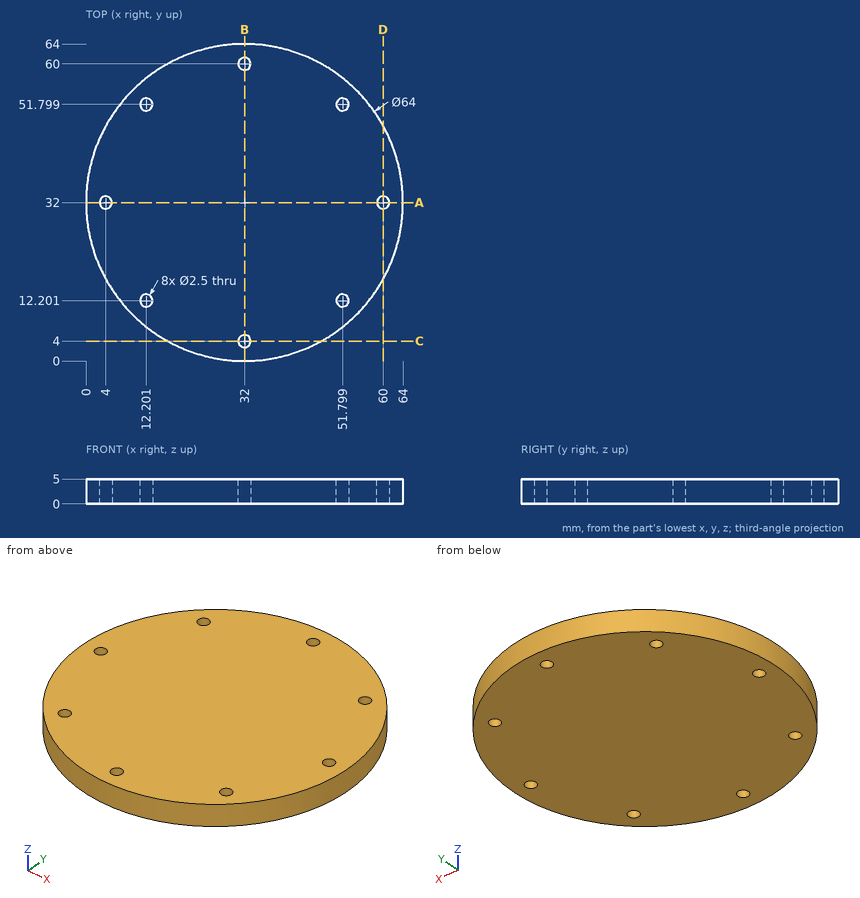
For this review, use the dimensioned drawing (mm, ordinates from the lowest corner) and the shaded views. Give positions to 0.01 mm unless a question says otherwise; leave off trailing zeros. Loops run counter-clockwise (first coordinate to the right, second up) from the corner with the lowest first, then second, coordinate; pieces in that order, holes last. Notation, with made-up numbers: (49, 53) -> (102, 53) arc R13 ccw to (102, 73) -> close; hole circle Ø5 at (68, 8). An arc over 180 degrees is marked (long way). Use CSV: the item, a comma, the result in double quotes.
1. To check wall thickness, follow probe 1 along Y at (x, z) = (32, 2.2); probe 2 along Y at (x, z) = (31, 2.1); probe 3 along X at (y, z) = (19, 4.7). State the ranges of each line that lie inside material, in increasing order. Write a range as from..to.
Result:
probe 1,"y = 0..2.75, 5.25..58.75, 61.25..64"
probe 2,"y = 0.02..3.25, 4.75..59.25, 60.75..63.98"
probe 3,"x = 2.76..61.24"
2. For P1, Ø1.5, axis at x = 24.5, z = 2, coming from the -Y side; P2, Ø3, axis at y = 53.5, z = 3.5, coming from the +X side; P3, Ø3, axis at y = 20, z = 3, coming from the +X side, all flat-tipped, find the tip position at first contact; note any pin that passes through.
Result:
P1,"stops at y = 0.72"
P2,"stops at x = 56.98"
P3,"stops at x = 62.23"
3. Consider section A-A, the plane y = 32. Write out the cut boundary in (x, z).
Result:
outline,"(0, 0) -> (2.75, 0) -> (2.75, 5) -> (0, 5) -> close; (5.25, 0) -> (58.75, 0) -> (58.75, 5) -> (5.25, 5) -> close; (61.25, 0) -> (64, 0) -> (64, 5) -> (61.25, 5) -> close"
4. Consider section C-C, the plane y = 4. Write out the cut boundary in (x, z), then the cut area to 3 significant figures.
Result:
outline,"(16.51, 0) -> (30.75, 0) -> (30.75, 5) -> (16.51, 5) -> close; (33.25, 0) -> (47.49, 0) -> (47.49, 5) -> (33.25, 5) -> close"
area,"142 mm²"
